```python
from build123d import *

# Parameters (mm, degrees)
F1_DEPTH = 13.14
F2_T     = -2.5


with BuildPart() as f1:
    # F0 (on Front) → F1 (new body)
    with BuildSketch(Plane.XZ):
        with BuildLine():
            Line((-18.325, -9.2), (15.325, -9.2))
            ThreePointArc((15.325, -9.2), (17.44632, -8.32132), (18.325, -6.2))
            Line((18.325, -6.2), (18.325, 6.2))
            ThreePointArc((18.325, 6.2), (17.44632, 8.32132), (15.325, 9.2))
            Line((15.325, 9.2), (-18.325, 9.2))
            Line((-18.325, 9.2), (-18.325, -9.2))
        make_face()
    extrude(amount=F1_DEPTH)

    # F2
    f2_openings = [f1.faces().sort_by_distance(p)[0] for p in [
        (-18.325, -6.57, 0),
    ]]
    offset(amount=F2_T, openings=f2_openings)


solid = f1.part
```
Work out the finished part from the listing and answer in its coordinate system (mm). A direction names the side the tool comes from. Round coordinates to 2 decimals unless told otherwise and drop trailing zeros. Write each loop counter-clockwise with the first axis right and the second up, starting at its lowest first coordinate (ties: lowest second). Pieces come first, ordered by that corner, then holes. Notation, with made-up numbers: (81, -27.5) -> (125, -27.5) arc R22 cw to (125, -11.5) -> close; hole circle Ø11 at (57, 19). An arc over 180 degrees is marked (long way). Write each question's results on one line, items separated by ' | '.
Q1. A flat-ended cylindrical pin translates along its axis: P1, Ø2, axis at y = -5, z = -1, coming from the -X side (3 decimals). Find the tip coordinate at first contact, or state that the pin passes through.
Data:
P1: x = 15.825
Q2. Section B-B, the plane y = -7.5 is taken. Write down the section's boundary in (x, z) (3 decimals).
Data:
outline: (-18.325, -9.2) -> (15.325, -9.2) arc R3 ccw to (18.325, -6.2) -> (18.325, 6.2) arc R3 ccw to (15.325, 9.2) -> (-18.325, 9.2) -> (-18.325, 6.7) -> (15.325, 6.7) arc R0.5 cw to (15.825, 6.2) -> (15.825, -6.2) arc R0.5 cw to (15.325, -6.7) -> (-18.325, -6.7) -> close
Q3. Section A-A, the plane x = -9 is taken. Write down the section's boundary in (y, z), then the cut area to 3 significant figures.
Data:
outline: (-13.14, -9.2) -> (0, -9.2) -> (0, 9.2) -> (-13.14, 9.2) -> close; hole (-10.64, -6.7) -> (-2.5, -6.7) -> (-2.5, 6.7) -> (-10.64, 6.7) -> close | area: 133 mm^2
Q4. Which of the six approach directions +Z, -Z, +X, -X, +Y, -Y give full straight-line access (tool end or side, diameter ignored) to faces 1 (the flat face through (-1, -2.5, 0)), 2 (the flat face through (0, 0, 0))?
Data:
face 1: -X | face 2: +Z, -Z, +X, -X, +Y
Q5. Straight lines are drawn through the part: line 1 along Y through (x, z) = (13, 1); line 2 along Z through (x, y) = (10, -2.75); line 3 along X through (y, z) = (-7.5, 2.5) (3 decimals). For each, find the intervals that lie inside material, in ascending order. Write a range as [from, to].
Data:
line 1: [-13.14, -10.64], [-2.5, 0] | line 2: [-9.2, -6.7], [6.7, 9.2] | line 3: [15.825, 18.325]
Q6. Determine the mould class of faces 3 (the flat face through (18.325, -6, 0)), 4 (the flat face through (0, -13.14, 0)), 5 (the flat face through (15.825, -7, 0)), 6 (the flat face through (-1, -7, 6.7)) for opening direction Y: released by +Y, released by -Y, zero draft, split by the parting line, or undercut.
Data:
face 3: zero draft | face 4: released by -Y | face 5: undercut | face 6: undercut
Q7. Section C-C, the plane z = 3.5 is taken. Write down the section's boundary in (x, y) (3 decimals), then the cut area to 3 significant figures.
Data:
outline: (-18.325, -13.14) -> (18.325, -13.14) -> (18.325, 0) -> (-18.325, 0) -> (-18.325, -2.5) -> (15.825, -2.5) -> (15.825, -10.64) -> (-18.325, -10.64) -> close | area: 204 mm^2
